Source: three-view drawing plus pictorial views. Frame: mm from the lowest corner of the part. A direction names the side the tool comes from. Round coordinates to 2 decimals unless told otherwise and drop trailing zeros. Write each loop counter-clockwise with the first axis right and the second up, starting at its lowest first coordinate (ties: lowest second). Pieces come first, ordered by that corner, then holes. Notation, with made-up numbers: (48, 44) -> (88, 44) arc R29 ccw to (88, 71) -> close; hole circle Ø1 at (9.25, -9). An arc over 180 degrees is marked (long way). Put each result on its own line as item: value.
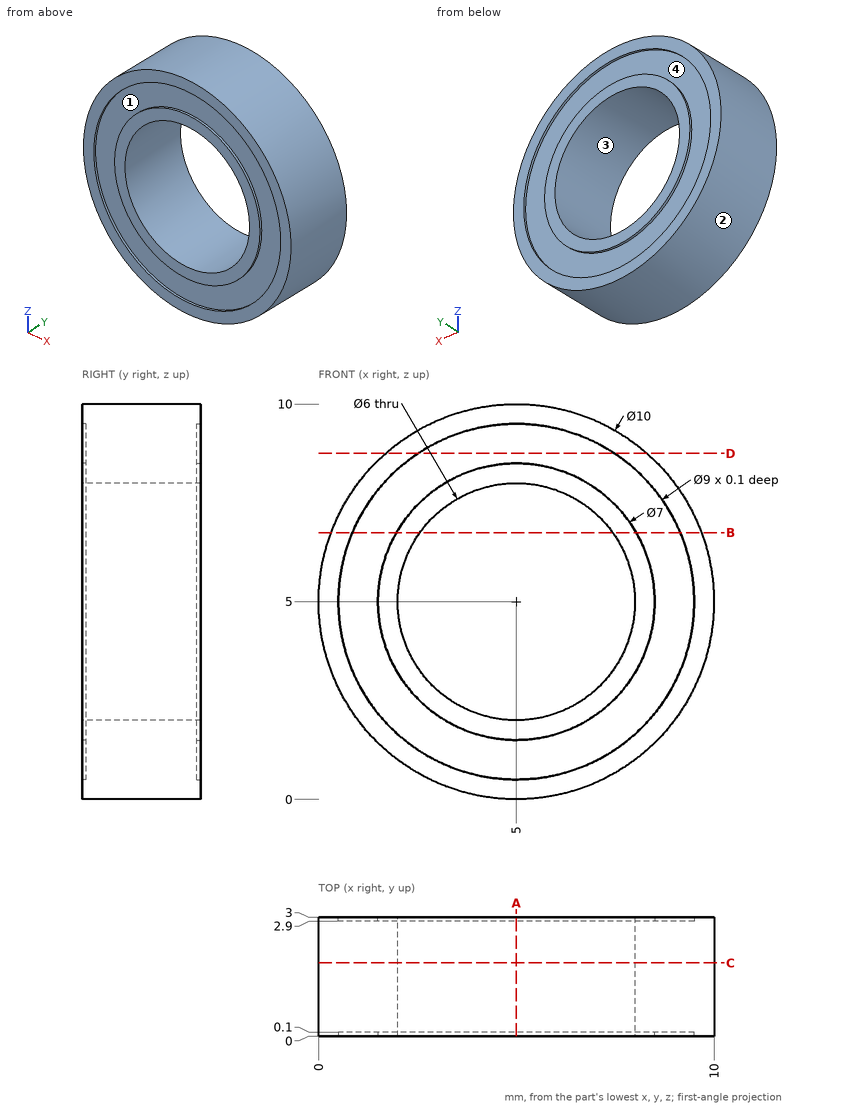
Q1. Cut plane B-B on z = 6.75. Output: boundary loops of the cut face in (x, y), and give its area (3 significant figures).
Ans:
outline: (0.32, 0) -> (0.85, 0) -> (0.85, 0.1) -> (1.97, 0.1) -> (1.97, 0) -> (2.56, 0) -> (2.56, 3) -> (1.97, 3) -> (1.97, 2.9) -> (0.85, 2.9) -> (0.85, 3) -> (0.32, 3) -> close; (7.44, 0) -> (8.03, 0) -> (8.03, 0.1) -> (9.15, 0.1) -> (9.15, 0) -> (9.68, 0) -> (9.68, 3) -> (9.15, 3) -> (9.15, 2.9) -> (8.03, 2.9) -> (8.03, 3) -> (7.44, 3) -> close
area: 13.0 mm^2
Q2. Cut plane A-A on x = 5. Output: boundary loops of the cut face in (y, z), and give its area (3 significant figures).
Ans:
outline: (0, 0) -> (3, 0) -> (3, 0.5) -> (2.9, 0.5) -> (2.9, 1.5) -> (3, 1.5) -> (3, 2) -> (0, 2) -> (0, 1.5) -> (0.1, 1.5) -> (0.1, 0.5) -> (0, 0.5) -> close; (0, 8) -> (3, 8) -> (3, 8.5) -> (2.9, 8.5) -> (2.9, 9.5) -> (3, 9.5) -> (3, 10) -> (0, 10) -> (0, 9.5) -> (0.1, 9.5) -> (0.1, 8.5) -> (0, 8.5) -> close
area: 11.6 mm^2
Q3. Cut plane C-C on y = 1.85. Output: boundary loops of the cut face in (x, z), and give its area (3 significant figures).
Ans:
outline: circle Ø10 at (5, 5); hole circle Ø6 at (5, 5)
area: 50.3 mm^2
Q4. Draft query along X for the marked faces 1 and 2. Return one class per face: +X half, -X half, draft (parallel to the pull), parting line (faces both ways), or undercut.
Ans:
face 1: undercut
face 2: parting line
Q5. Cut plane D-D on z = 8.75. Output: boundary loops of the cut face in (x, y), and give its area (3 significant figures).
Ans:
outline: (1.69, 0) -> (2.51, 0) -> (2.51, 0.1) -> (7.49, 0.1) -> (7.49, 0) -> (8.31, 0) -> (8.31, 3) -> (7.49, 3) -> (7.49, 2.9) -> (2.51, 2.9) -> (2.51, 3) -> (1.69, 3) -> close
area: 18.8 mm^2
Q6. Material intervals for line 1 (Z direction, x = 5, y = 2.95); line 2 (Z direction, x = 5, y = 2.35); line 3 (Y direction, x = 2.75, z = 8.25), sorted ascending. Write a range as [from, to].
Ans:
line 1: z = [0, 0.5], [1.5, 2], [8, 8.5], [9.5, 10]
line 2: z = [0, 2], [8, 10]
line 3: y = [0.1, 2.9]
Q7. Pin query (flat end, axial travel): pin 1 (2.5 mm diameter, centred on x = 6, z = 5, fed in from +Y); pin 2 (1.5 mm diameter, centred on x = 1, y = 2, fed in from +Z). Return the tip coordinate at first contact, or that it passes through.
Ans:
pin 1: passes through
pin 2: stops at z = 8.8
Q8. Reachability of the marked faces 3 and 4 from +Z, -Z, +X, -X, +Y, -Y: full face, straight path, thin tool, end or side. Return the list, or none.
Ans:
face 3: +Y, -Y
face 4: +Y
